Model file for the job. Use its own axes, mm. A direction names the side the tool comes from. Coordinates: 2 decimals unless noted, no trailing zeros. Write each loop counter-clockwise with the first axis right and the second up, starting at its lowest first coordinate (ties: lowest second). Pieces come first, ordered by that corner, then holes. Notation, with made-up numbers: (81.25, 71) - (87.25, 71) arc R17 ccw to (87.25, 85) - close; hole circle Ø8 at (-29, 88). An arc over 180 degrees is marked (long way). Put each result on its own line as item: value. Start each with the question number.
1. Drill centre lines: L1, parallel to X at y = 148, z = 6.5; L2, parallel to Z at x = 106, y = 184; L3, parallel to Y at x = -106, z = 0. Where is each one in solid material? Low to high. Write a range as from..to.
2. Drop flat-ended pins along their axis: P1, Ø2, axis at x = 34.5, z = 1.5, coming from the +Y side; P2, Ø20.5, axis at y = 184.15, z = 0, coming from the +X side. Give the stop position or say it passes through.
3. Saw through at C-C, the plane z = -6.5. Write the cut outline in (x, y), plus the area to 3 significant figures.
4. Saw through at A-A, the plane y = 110. Write the cut outline in (x, z), plus the area to 3 significant figures.
5. Saw through at D-D, the plane x = -38.5. Write the cut outline in (y, z).
6. Saw through at B-B, the plane y = 184.15. Write the cut outline in (x, z), plus the area to 3 significant figures.
7. Pull direction Z, two halves, no side cores. Call faces 3 (the face through (2, -6.35, 0)), 4 (the face through (17, -2, -19.05)), 5 (the face through (-108.04, 171.75, -2.75)): released by +Z, released by -Z, zero draft, split by the parting line, or undercut.
8. Which spindle directions (+Z, -Z, +X, -X, +Y, -Y) get a long thin tool onto all of the face, cutting with end or side? Do faces 1 (the face through (108, 203.2, 0)), 2 (the face through (87.114, 15.276, -0.267)). Say none if no direction does.
Autodesk Inventor part; units mm, degrees
ref_plane "YZ Plane" through (0, 0, 0) normal (1, 0, 0) x (0, 1, 0)
ref_plane "XZ Plane" through (0, 0, 0) normal (0, 1, 0) x (-1, 0, 0)
ref_plane "XY Plane" through (0, 0, 0) normal (0, 0, 1) x (1, 0, 0)
sketch "Sketch1" plane through (0, 0, 0) normal (0, 1, 0) x (-1, 0, 0)
  line L0 (114.3, 19.05) -> (-114.3, 19.05)
  line L1 (-114.3, 19.05) -> (-114.3, -19.05)
  line L2 (-114.3, -19.05) -> (114.3, -19.05)
  line L3 (114.3, -19.05) -> (114.3, 19.05)
  line L4 (114.3, 19.05) -> (-114.3, -19.05) construction
  line L5 (-114.3, 19.05) -> (114.3, -19.05) construction
  point P0 (0, 0)
  dimension "d0" = 228.6
  dimension "d1" = 38.1
extrude "Extrusion1" add sketch "Sketch1" against normal blind 6.35
sketch "Sketch2" plane through (0, 0, 0) normal (0, 1, 0) x (1, 0, 0)
  line L0 (-114.3, -19.05) -> (-114.3, 19.05)
  line L1 (-114.3, 19.05) -> (114.3, 19.05)
  line L2 (-114.3, -19.05) -> (-101.6, -19.05)
  line L3 (-101.6, -19.05) -> (-101.6, 19.05)
  line L4 (-101.6, 19.05) -> (-114.3, 19.05)
  line L5 (-114.3, 19.05) -> (-114.3, -19.05)
  line L6 (114.3, 19.05) -> (114.3, -19.05)
  line L7 (114.3, -19.05) -> (101.6, -19.05)
  line L8 (101.6, -19.05) -> (101.6, 19.05)
  line L9 (101.6, 19.05) -> (114.3, 19.05)
  line L10 (114.3, 19.05) -> (114.3, -19.05)
  point P0 (0, 0)
  dimension "d4" = 12.7
  dimension "d5" = 12.7
extrude "Extrusion2" add sketch "Sketch2" along normal blind 203.2
sketch "Sketch3" plane through (-114.3, -6.35, -19.05) normal (-1, 0, 0) x (0, 0, 1)
  line L0 (0, 209.55) -> (38.1, 209.55) construction
  line L1 (19.05, 209.55) -> (19.05, 0) construction
  line L2 (38.1, 0) -> (0, 0) construction
  circle A0 centre (19.05, 190.5) radius 12.7
  line L3 (0, 6.35) -> (0, 209.55) construction
  line L4 (0, 203.2) -> (38.1, 203.2) construction
  point P0 (19.05, 6.35)
  dimension "d8" = 25.4
  dimension "d9" = 6.35
extrude "Extrusion3" cut sketch "Sketch3" against normal through all
fillet "Fillet1" radius 50.8 2 edges at (101.6, 0, 0) (-101.6, 0, 0)
properties part number "fork04"
Final values:
1. L1: x = -114.3..-101.6, 101.6..114.3
1. L2: z = -19.05..-12.7, 12.7..19.05
1. L3: y = -6.35..171.45, 196.85..203.2
2. P1: stops at y = 0
2. P2: passes through
3. outline: (-114.3, -6.35) - (114.3, -6.35) - (114.3, 173.24) - (101.6, 173.24) - (101.6, 50.8) arc R50.8 cw to (50.8, 0) - (-50.8, 0) arc R50.8 cw to (-101.6, 50.8) - (-101.6, 173.24) - (-114.3, 173.24) - close; (-114.3, 195.06) - (-101.6, 195.06) - (-101.6, 203.2) - (-114.3, 203.2) - close; (101.6, 195.06) - (114.3, 195.06) - (114.3, 203.2) - (101.6, 203.2) - close
3. area: 7,170 mm²
4. outline: (-114.3, -19.05) - (-101.6, -19.05) - (-101.6, 19.05) - (-114.3, 19.05) - close; (101.6, -19.05) - (114.3, -19.05) - (114.3, 19.05) - (101.6, 19.05) - close
4. area: 968 mm²
5. outline: (-6.35, -19.05) - (0, -19.05) - (0, 19.05) - (-6.35, 19.05) - close
6. outline: (-114.3, -19.05) - (-101.6, -19.05) - (-101.6, -12.7) - (-114.3, -12.7) - close; (-114.3, 12.7) - (-101.6, 12.7) - (-101.6, 19.05) - (-114.3, 19.05) - close; (101.6, -19.05) - (114.3, -19.05) - (114.3, -12.7) - (101.6, -12.7) - close; (101.6, 12.7) - (114.3, 12.7) - (114.3, 19.05) - (101.6, 19.05) - close
6. area: 323 mm²
7. face 3: zero draft
7. face 4: released by -Z
7. face 5: undercut
8. face 1: +Z, -Z, +X, -X, +Y
8. face 2: +Z, -Z, +Y
